Read the model definition and answer for the solid it produces. Units are mm, in the model's axes. Face numbers are marked on the shaded views. A direction names the side the tool comes from. Give positions to 0.01 mm unless a question says otherwise; leave off trailing zeros. Loops run counter-clockwise (first coordinate to the right, second up) from the corner with the lowest first, then second, coordinate; pieces in that order, holes last. Notation, with made-up numbers: (-36.75, 84) - (-13.75, 84) arc R12 ccw to (-13.75, 90) - close; hole circle Ø4 at (-39.5, 59). An arc over 180 degrees is marked (long way). Write item = value, one per line.
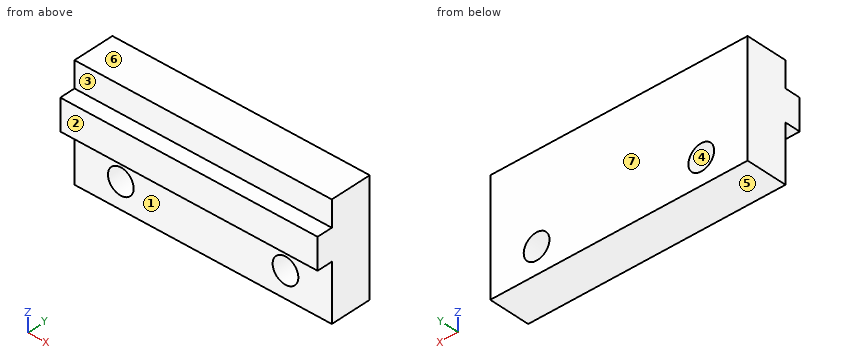
```python
from build123d import *

# Parameters (mm, degrees)
SKETCH1_W           = 25
SKETCH1_H           = 5
SKETCH1_R           = 1.25
BOSS_EXTRUDE1_DEPTH = 4
SKETCH2_W           = 25
SKETCH2_H           = 4
BOSS_EXTRUDE2_DEPTH = 6
SKETCH3_W           = 25
SKETCH3_H           = 3
BOSS_EXTRUDE3_DEPTH = 1.5


with BuildPart() as part:
    # Sketch1 → Boss-Extrude1 (new body)
    with BuildSketch(Plane(origin=(0, 0, 0), x_dir=(1, 0, 0), z_dir=(0, 1, 0))):
        with Locations((12.5, 2.5)):
            Rectangle(SKETCH1_W, SKETCH1_H)
        with Locations(Location((4.5, 2.5, 0), (0, 0, 270))):
            Circle(SKETCH1_R, mode=Mode.SUBTRACT)
        with Locations(Location((20.5, 2.5, 0), (0, 0, 270))):
            Circle(SKETCH1_R, mode=Mode.SUBTRACT)
    extrude(amount=BOSS_EXTRUDE1_DEPTH)

    # Sketch2 → Boss-Extrude2 (add)
    with BuildSketch(Plane.XY):
        with Locations((12.5, 2)):
            Rectangle(SKETCH2_W, SKETCH2_H)
    extrude(amount=BOSS_EXTRUDE2_DEPTH)

    # Sketch3 → Boss-Extrude3 (add)
    with BuildSketch(Plane.XZ):
        with Locations((12.5, 2)):
            Rectangle(SKETCH3_W, SKETCH3_H)
    extrude(amount=BOSS_EXTRUDE3_DEPTH)


solid = part.part
```
1) A tool of negligible diameter and unlimited length cuts with its end or side. For the marked faces 1, 2 and 3, from which of +Z, -Z, +X, -X, +Y, -Y can it reach the whole face along a straight path? Write none if from no direction.
Output:
face_1 = -Z, +X, -X, -Y
face_2 = +Z, -Z, +X, -X, -Y
face_3 = +Z, +X, -X, -Y
2) Each of these flat-tipped pins is pushed along its axis until it touches: P1, Ø1.2, axis at x = 13, y = -0.5, coming from the +Z side; P2, Ø2, axis at x = 20.5, z = -2.5, coming from the -Y side. Where does it stop, or does it pass through?
Output:
P1 = 6
P2 = through
3) A cutting plane is placed at D-D on x = 12. Determine the outline of the cut face in (y, z).
Output:
outline = (-1.5, 0.5) - (0, 0.5) - (0, -5) - (4, -5) - (4, 6) - (0, 6) - (0, 3.5) - (-1.5, 3.5) - close
4) A cutting plane is placed at B-B on x = 4.25. Determine the outline of the cut face in (y, z), then the cut area to 3 significant figures.
Output:
outline = (-1.5, 0.5) - (0, 0.5) - (0, -1.28) - (4, -1.28) - (4, 6) - (0, 6) - (0, 3.5) - (-1.5, 3.5) - close; (0, -5) - (4, -5) - (4, -3.72) - (0, -3.72) - close
area = 38.7 mm²
5) A cutting plane is placed at A-A on z = -2.5. Determine the outline of the cut face in (x, y).
Output:
outline = (0, 0) - (3.25, 0) - (3.25, 4) - (0, 4) - close; (5.75, 0) - (19.25, 0) - (19.25, 4) - (5.75, 4) - close; (21.75, 0) - (25, 0) - (25, 4) - (21.75, 4) - close
6) The mould has two halves that part along Z. Classify the marked faces 4, 5, 6 and 7: pulls with the +Z half, pulls with the -Z half, needs draft (parallel to the pull), parting line crosses it, or undercut.
Output:
face_4 = undercut
face_5 = pulls with the -Z half
face_6 = pulls with the +Z half
face_7 = needs draft
7) A cutting plane is placed at C-C on y = 0.65. Determine the outline of the cut face in (x, z).
Output:
outline = (0, -5) - (25, -5) - (25, 6) - (0, 6) - close; hole circle Ø2.5 at (4.5, -2.5); hole circle Ø2.5 at (20.5, -2.5)
8) Find the intervals of material crossed by probe 1 along X at (y, z) = (2.9, -2.5); probe 2 along Z at (x, y) = (9, -0.25); probe 3 along Y at (x, z) = (6.5, -1.5), in increasing order.
Output:
probe_1 = 0 to 3.25, 5.75 to 19.25, 21.75 to 25
probe_2 = 0.5 to 3.5
probe_3 = 0 to 4
